Could you check a few things on this model? Use its own coordinates, in mm. Coordinates: 2 decimals unless noted, no trailing zeros. Order: outer loops, then holes, each group sorted by start corner. A loop starts at its lowest first (then second) coordinate and runs counter-clockwise, first axis right, second up. Notation, with made-up numbers: (-9.75, -7.5) -> (36.25, -7.5) arc R28 cw to (36.25, 21.5) -> close; hole circle Ø7 at (79.25, 7.25). An arc over 180 degrees is marked (long way). Put each result on its own line as item: value. Start each with the question number.
Q1. If we section it at B-B (z = 21.5): Please give me the cut outline in (x, y).
Q2. We'd pull the mould along X, two halves only. Please class faces 1 (the face through (0, 0, 9)), 2 (the face through (0, 0, 0)), 3 (the face through (-4.036, 30.736, 29.087)): +X half, -X half, draft (parallel to the pull), parting line (faces both ways), or undercut.
Q3. If we section it at D-D (y = -26): Please give me the cut outline in (x, z).
Q4. Will these pins go through, and if not, where does the flat tip stop? pin 1 (8 mm diameter, centred on x = -11.5, z = 6.5, fed in from +Y); pin 2 (6 mm diameter, centred on x = 17, z = 50.5, fed in from -Y); pin 3 (1 mm diameter, centred on y = -17, z = 14, fed in from +X); pin 4 (2 mm diameter, centred on x = 9, y = -21, fed in from +Z).
Q5. If we section it at C-C (y = 2): Please give me the cut outline in (x, z).
Q6. Please list where these lines run through material, in increasing order: line 1 along X through (y, z) = (-19, 27.5); line 2 along Z through (x, y) = (8, 13); line 3 along Y through (x, z) = (-2, 35).
Q7. If we section it at A-A (x = 16): Please give me the cut outline in (y, z).
from build123d import *

# Parameters (mm, degrees)
F0_R     = 31
F1_DEPTH = 59
F2_DEPTH = 9


with BuildPart() as f1:
    # F0 (on Top) → F1 (new body)
    with BuildSketch(Plane.XY):
        Circle(F0_R)
        with BuildLine():
            ThreePointArc((0, 23), (16.263456, 16.263456), (23, 0))
            ThreePointArc((23, 0), (16.263456, -16.263456), (0, -23))
            ThreePointArc((0, -23), (-23, 0), (0, 23))
        make_face(mode=Mode.SUBTRACT)
    extrude(amount=F1_DEPTH)

    # F0 (on Top) → F2 (join)
    with BuildSketch(Plane.XY):
        with BuildLine():
            Line((0, -23), (0, 23))
            ThreePointArc((0, 23), (-23, 0), (0, -23))
        make_face()
        with BuildLine():
            ThreePointArc((0, -23), (16.263456, -16.263456), (23, 0))
            ThreePointArc((23, 0), (16.263456, 16.263456), (0, 23))
            Line((0, 23), (0, -23))
        make_face()
    extrude(amount=F2_DEPTH)


solid = f1.part
The answers:
1. outline: circle Ø62 at (0, 0); hole circle Ø46 at (0, 0)
2. face 1: undercut
2. face 2: draft
2. face 3: parting line
3. outline: (-16.88, 0) -> (16.88, 0) -> (16.88, 59) -> (-16.88, 59) -> close
4. pin 1: y = 30.08
4. pin 2: y = -27.66
4. pin 3: x = 26.24
4. pin 4: z = 59
5. outline: (-30.94, 0) -> (30.94, 0) -> (30.94, 59) -> (22.91, 59) -> (22.91, 9) -> (-22.91, 9) -> (-22.91, 59) -> (-30.94, 59) -> close
6. line 1: -24.49 to -12.96, 12.96 to 24.49
6. line 2: 0 to 9
6. line 3: -30.94 to -22.91, 22.91 to 30.94
7. outline: (-26.55, 0) -> (26.55, 0) -> (26.55, 59) -> (16.52, 59) -> (16.52, 9) -> (-16.52, 9) -> (-16.52, 59) -> (-26.55, 59) -> close
